Verification items for the finished model (mm, model axes). A direction names the side the tool comes from. Give positions to 0.01 mm unless a question says otherwise; leave off trailing zeros. Loops run counter-clockwise (first coordinate to the right, second up) from the corner with the lowest first, then second, coordinate; pieces in that order, holes last. Notation, with made-up numbers: (33, 84.5) - (44, 84.5) arc R9 cw to (44, 89.5) - close; hole circle Ø4 at (-5.75, 61). An arc over 180 degrees is marked (long way). One line per item, written item: value. Start each with the question number.
1. Sectioned sample at A-A (y = 15). Record the cut outline in (x, z), plus the area to 3 significant figures.
2. Scan lines: L1, parallel to X at y = 3.5, z = 26.5; L2, parallel to X at y = 41.5, z = 12; L3, parallel to X at y = -1.5, z = -20.5. Record each from-to range of solid material in increasing order. Write a range as [from, to].
3. Access from +Z, -Z, +X, -X, +Y, -Y to the whole of each face (thin tool, end or side, straight path). Record for faces 1 (the flat face through (-108, 8.986, 21)), 2 (the flat face through (-150.738, 22.721, 27.772)), 3 (the flat face through (-155, 32.313, 14)), 4 (the flat face through (-153, 32.313, -27)).
4. Sectioned sample at B-B (y = 35). Record the cut outline in (x, z).
5. Mould release check, pull along X, two halves, no side actions. Record for faces 5 (the flat face through (-151.15, 22.72, -25.46)), 6 (the flat face through (-151.13, 22.72, -27.85)), 7 (the flat face through (-107, 0, -21)): pulls with the +X half, pulls with the -X half, needs draft (parallel to the pull), parting line crosses it, or undercut.
6. Gauge pin test, flat ends, axial feed: pin 1 (12 mm diameter, centred on y = 35.5, z = -14.5, fed in from +X); pin 2 (2 mm diameter, centred on y = 8.5, z = -13, fed in from +X); pin 3 (2.5 mm diameter, centred on x = -150, z = -27, fed in from +Y); pin 4 (5 mm diameter, centred on x = -121, y = 1, fed in from -Z) (1 decimal). Record the tip position at first contact, or that the pin passes through.
from build123d import *

# Parameters (mm, degrees)
REVOLVE1_ANGLE                  = 15
REVOLVE1_OTHER_WAY_ANGLE        = 15
REVOLVE2_START                  = 16.222144695
REVOLVE2_DEPTH                  = 16.090427574
CIRPATTERN1_COUNT               = 3
CIRPATTERN1_ANGLE               = 10
CIRPATTERN1_THE_OTHER_WAY_COUNT = 3
CIRPATTERN1_THE_OTHER_WAY_ANGLE = 10
SHELL3_START                    = 8.985762726
SHELL3_2_DEPTH                  = 42.380509533
SHELL3_START_2                  = 17.722144695
SHELL3_3_DEPTH                  = 13.090427574
SKETCH3_W                       = 5.112055803
SKETCH3_H                       = 7.485762726
REVOLVE3_ANGLE                  = 15
REVOLVE3_OTHER_WAY_ANGLE        = 15
CUT_REVOLVE2_ANGLE              = 7
CUT_REVOLVE2_OTHER_WAY_ANGLE    = 7
SKETCH11_R                      = 2


with BuildPart() as part:
    # Sketch1 → Revolve1 (revolve)
    with BuildSketch(Plane.XY):
        with BuildLine():
            Line((-111.783895357, 7.485762726), (-118.250728673, -4.885300025))
            ThreePointArc((-118.250728673, -4.885300025), (-124.705004152, -9.547595462), (-132.307869355, -7.183042355))
            ThreePointArc((-132.307869355, -7.183042355), (-138.813052314, -0.732302942), (-145.106903203, 5.924789912))
            ThreePointArc((-145.106903203, 5.924789912), (-154.580954265, 28.121202409), (-148.092110072, 51.366272259))
            Line((-148.092110072, 51.366272259), (-106.671839554, 51.366272259))
            Line((-106.671839554, 51.366272259), (-106.671839554, 7.485762726))
            Line((-106.671839554, 7.485762726), (-111.783895357, 7.485762726))
        make_face()
    revolve(axis=Axis((0, 75.962527062, 0), (0, -1, 0)), revolution_arc=REVOLVE1_ANGLE)

    # Sketch1 → Revolve1 other way (revolve)
    with BuildSketch(Plane.XY):
        with BuildLine():
            Line((-111.783895357, 7.485762726), (-118.250728673, -4.885300025))
            ThreePointArc((-118.250728673, -4.885300025), (-124.705004152, -9.547595462), (-132.307869355, -7.183042355))
            ThreePointArc((-132.307869355, -7.183042355), (-138.813052314, -0.732302942), (-145.106903203, 5.924789912))
            ThreePointArc((-145.106903203, 5.924789912), (-154.580954265, 28.121202409), (-148.092110072, 51.366272259))
            Line((-148.092110072, 51.366272259), (-106.671839554, 51.366272259))
            Line((-106.671839554, 51.366272259), (-106.671839554, 7.485762726))
            Line((-106.671839554, 7.485762726), (-111.783895357, 7.485762726))
        make_face()
    revolve(axis=Axis((0, 75.962527062, 0), (0, 1, 0)), revolution_arc=REVOLVE1_OTHER_WAY_ANGLE)

    # Revolve2: read off the stored shape, not the designer's step
    # Revolve2 outline → Revolve2 (add)
    with BuildSketch(Plane(origin=(0, 0, 0), x_dir=(1, 0, 0), z_dir=(0, 1, 0)).offset(REVOLVE2_START)):
        with BuildLine():
            ThreePointArc((-156.32174005, 2.728606122), (-156.345552235, 0), (-156.32174005, -2.728606122))
            Line((-156.32174005, -2.728606122), (-151.716418742, -2.64821994))
            Line((-151.716418742, -2.64821994), (-150, -2.61825974))
            Line((-150, -2.61825974), (-150, 2.61825974))
            Line((-150, 2.61825974), (-151.716418742, 2.64821994))
            Line((-151.716418742, 2.64821994), (-156.32174005, 2.728606122))
        make_face()
    revolve2 = extrude(amount=REVOLVE2_DEPTH)

    # CirPattern1: Revolve2 ×3 about axis
    cirpattern1_axis = Axis((0, 0, 0), (0, 1, 0))
    for i in range(1, CIRPATTERN1_COUNT):
        add(revolve2.rotate(cirpattern1_axis, i * CIRPATTERN1_ANGLE / (CIRPATTERN1_COUNT - 1)))

    # CirPattern1 the other way: Revolve2 ×3 about axis
    cirpattern1_the_other_way_axis = Axis((0, 0, 0), (0, -1, 0))
    for i in range(1, CIRPATTERN1_THE_OTHER_WAY_COUNT):
        add(revolve2.rotate(cirpattern1_the_other_way_axis, i * CIRPATTERN1_THE_OTHER_WAY_ANGLE / (CIRPATTERN1_THE_OTHER_WAY_COUNT - 1)))

    # Shell3: read off the stored shape, not the designer's step
    # Shell3 outline → Shell3 (revolve, cut)
    with BuildSketch(Plane.XY):
        with BuildLine():
            ThreePointArc((131.268982929, -6.101046516), (137.739825777, 0.315640187), (144.000452154, 6.937591016))
            ThreePointArc((144.000452154, 6.937591016), (153.114903986, 28.748570347), (146.242378119, 51.366272259))
            Line((146.242378119, 51.366272259), (112.692366824, 51.366272259))
            Line((112.692366824, 51.366272259), (112.692366824, 8.985762726))
            Line((112.692366824, 8.985762726), (119.5800606, -4.190406776))
            ThreePointArc((119.5800606, -4.190406776), (124.946978842, -8.067241366), (131.268982929, -6.101046516))
        make_face()
    revolve(axis=Axis((0, 0, 0), (0, 1, 0)), mode=Mode.SUBTRACT)

    # Shell3 2 outline → Shell3 2 (cut)
    with BuildSketch(Plane(origin=(0, 0, 0), x_dir=(1, 0, 0), z_dir=(0, 1, 0)).offset(SHELL3_START)):
        with BuildLine():
            Line((-103.037084763, 27.608703653), (-108.852467541, 29.166930772))
            ThreePointArc((-108.852467541, 29.166930772), (-112.692366824, 0), (-108.852467541, -29.166930772))
            Line((-108.852467541, -29.166930772), (-103.037084763, -27.608703653))
            ThreePointArc((-103.037084763, -27.608703653), (-106.671839554, 0), (-103.037084763, 27.608703653))
        make_face()
    extrude(amount=SHELL3_2_DEPTH, mode=Mode.SUBTRACT)

    # Shell3 3 outline → Shell3 3 (cut)
    with BuildSketch(Plane(origin=(0, 0, 0), x_dir=(1, 0, 0), z_dir=(0, 1, 0)).offset(SHELL3_START_2)):
        with BuildLine():
            ThreePointArc((-154.840882749, 1.20252917), (-154.845552235, 0), (-154.840882749, -1.20252917))
            Line((-154.840882749, -1.20252917), (-150.729272176, -1.13076074))
            Line((-150.729272176, -1.13076074), (-112.691399989, -0.466807206))
            ThreePointArc((-112.691399989, -0.466807206), (-112.692366824, 0), (-112.691399989, 0.466807206))
            Line((-112.691399989, 0.466807206), (-150.729272176, 1.13076074))
            Line((-150.729272176, 1.13076074), (-154.840882749, 1.20252917))
        make_face()
        with BuildLine():
            ThreePointArc((-112.22189026, -10.286733541), (-112.263538345, -9.821786937), (-112.303260118, -9.356671802))
            Line((-112.303260118, -9.356671802), (-150.254254081, -12.010463816))
            Line((-150.254254081, -12.010463816), (-154.356473766, -12.29731896))
            ThreePointArc((-154.356473766, -12.29731896), (-154.25631816, -13.495679116), (-154.14685912, -14.693225327))
            Line((-154.14685912, -14.693225327), (-150.057149497, -14.263379525))
            Line((-150.057149497, -14.263379525), (-112.22189026, -10.286733541))
        make_face()
        with BuildLine():
            Line((-150.254254081, 12.010463816), (-112.303260118, 9.356671802))
            ThreePointArc((-112.303260118, 9.356671802), (-112.263538345, 9.821786937), (-112.22189026, 10.286733541))
            Line((-112.22189026, 10.286733541), (-150.057149497, 14.263379525))
            Line((-150.057149497, 14.263379525), (-154.14685912, 14.693225327))
            ThreePointArc((-154.14685912, 14.693225327), (-154.25631816, 13.495679116), (-154.356473766, 12.29731896))
            Line((-154.356473766, 12.29731896), (-150.254254081, 12.010463816))
        make_face()
        with BuildLine():
            ThreePointArc((-110.898304185, -20.028371609), (-110.980316554, -19.568824134), (-111.060424629, -19.108940881))
            Line((-111.060424629, -19.108940881), (-148.635710387, -25.06028149))
            Line((-148.635710387, -25.06028149), (-152.697318814, -25.703577068))
            ThreePointArc((-152.697318814, -25.703577068), (-152.493100361, -26.888647965), (-152.279684816, -28.072097167))
            Line((-152.279684816, -28.072097167), (-110.898304185, -20.028371609))
        make_face()
        with BuildLine():
            Line((-148.635710387, 25.06028149), (-111.060424629, 19.108940881))
            ThreePointArc((-111.060424629, 19.108940881), (-110.980316554, 19.568824134), (-110.898304185, 20.028371609))
            Line((-110.898304185, 20.028371609), (-152.279684816, 28.072097167))
            ThreePointArc((-152.279684816, 28.072097167), (-152.493100361, 26.888647965), (-152.697318814, 25.703577068))
            Line((-152.697318814, 25.703577068), (-148.635710387, 25.06028149))
        make_face()
    extrude(amount=SHELL3_3_DEPTH, mode=Mode.SUBTRACT)

    # Sketch3 → Revolve3 (revolve)
    with BuildSketch(Plane.XY):
        with Locations((-109.227867456, 3.742881363)):
            Rectangle(SKETCH3_W, SKETCH3_H)
    revolve(axis=Axis((0, 7.485762726, 0), (0, 1, 0)), revolution_arc=REVOLVE3_ANGLE)

    # Sketch3 → Revolve3 other way (revolve)
    with BuildSketch(Plane.XY):
        with Locations((-109.227867456, 3.742881363)):
            Rectangle(SKETCH3_W, SKETCH3_H)
    revolve(axis=Axis((0, 7.485762726, 0), (0, -1, 0)), revolution_arc=REVOLVE3_OTHER_WAY_ANGLE)

    # Sketch8 → Cut-Revolve2 (revolve, cut)
    with BuildSketch(Plane.XY):
        with BuildLine():
            Line((-124.705004152, -9.547595462), (-130.523628013, 26.049613644))
            Line((-130.523628013, 26.049613644), (-106.671839554, 29.948362701))
            Line((-106.671839554, 29.948362701), (-106.671839554, 7.485762726))
            Line((-106.671839554, 7.485762726), (-106.671839554, 0))
            Line((-106.671839554, 0), (-111.783895357, 0))
            Line((-111.783895357, 0), (-111.783895357, 7.485762726))
            Line((-111.783895357, 7.485762726), (-118.250728673, -4.885300025))
            ThreePointArc((-118.250728673, -4.885300025), (-120.927677668, -7.978104694), (-124.705004152, -9.547595462))
        make_face()
    revolve(axis=Axis((0, 7.485762726, 0), (0, 1, 0)), revolution_arc=CUT_REVOLVE2_ANGLE, mode=Mode.SUBTRACT)

    # Sketch8 → Cut-Revolve2 other way (revolve, cut)
    with BuildSketch(Plane.XY):
        with BuildLine():
            Line((-124.705004152, -9.547595462), (-130.523628013, 26.049613644))
            Line((-130.523628013, 26.049613644), (-106.671839554, 29.948362701))
            Line((-106.671839554, 29.948362701), (-106.671839554, 7.485762726))
            Line((-106.671839554, 7.485762726), (-106.671839554, 0))
            Line((-106.671839554, 0), (-111.783895357, 0))
            Line((-111.783895357, 0), (-111.783895357, 7.485762726))
            Line((-111.783895357, 7.485762726), (-118.250728673, -4.885300025))
            ThreePointArc((-118.250728673, -4.885300025), (-120.927677668, -7.978104694), (-124.705004152, -9.547595462))
        make_face()
    revolve(axis=Axis((0, 7.485762726, 0), (0, -1, 0)), revolution_arc=CUT_REVOLVE2_OTHER_WAY_ANGLE, mode=Mode.SUBTRACT)

    # Sketch11 → Cut-Revolve3 (revolve, cut)
    with BuildSketch(Plane(origin=(0, 0, 0), x_dir=(0.9659258262890682, 0, -0.25881904510252135), z_dir=(0.2588190451025213, 0, 0.9659258262890681)), mode=Mode.PRIVATE) as cut_revolve3_sk:
        with Locations((-109.377957305, 3.882584066)):
            Circle(SKETCH11_R)
    revolve(cut_revolve3_sk.sketch.rotate(Axis((0, 7.485762726, 0), (0, 1, 0)), 334), axis=Axis((0, 7.485762726, 0), (0, 1, 0)), mode=Mode.SUBTRACT)


solid = part.part
Results are:
1. outline: (-146.04, -39.13) - (-144.43, -38.7) arc R149.53 cw to (-144.43, 38.7) - (-146.04, 39.13) arc R151.19 ccw to start
1. area: 131 mm^2
2. L1: x = [-140.38, -138.28], [-112.48, -110.74], [-108.6, -108.14], [-104.09, -103.33]
2. L2: x = [-152.49, -150.91]
2. L3: x = [-136.53, -134.4], [-116.38, -114.66]
3. face 1: +Z, -Z, +X, +Y
3. face 2: none
3. face 3: +Z, -X, +Y
3. face 4: -Z, -X, +Y
4. outline: (-149.12, -39.96) - (-147.66, -39.57) arc R152.87 cw to (-147.66, 39.57) - (-149.12, 39.96) arc R154.38 ccw to start
5. face 5: pulls with the +X half
5. face 6: undercut
5. face 7: needs draft
6. pin 1: stops at x = -150.59
6. pin 2: stops at x = -105.75
6. pin 3: stops at y = 46.08
6. pin 4: passes through
